Could you check a few things on this model? Use its own coordinates, in mm. A direction names the side the tool comes from. Round coordinates to 2 decimals unless told otherwise and drop trailing zeros. Write each loop counter-clockwise with the first axis right and the second up, starting at its lowest first coordinate (ties: lowest second). Pieces come first, ordered by that corner, then holes. Notation, with made-up numbers: (-8.75, 45.5) -> (29.25, 45.5) arc R34 cw to (29.25, 77.5) -> close; hole circle Ø7 at (62, 23.5). An arc over 180 degrees is marked (long way). Answer as CSV lines item,"result". Start each with the question number.
Q1. If I drill on line 1 (Y direction, x = 3.25, z = -2.5); line 2 (Y direction, x = -1.5, z = -2); line 3 (X direction, y = 4.5, z = 4), over which ranges is the centre line in solid material (lowest first)? Write a range as [from, to].
Q2. Imagine slicing it at A-A on z = 0. Please give me the cut outline in (x, y).
Q3. Imagine slicing it at B-B on x = 0. Please give me the cut outline in (y, z).
Q4. Imagine slicing it at C-C on y = 16.5. Please give me the cut outline in (x, z), and give its area (3 significant figures).
Q5. Will these pins go through, and if not, where does the flat tip stop? pin 1 Ø1.5 at (x, y) = (-1.5, 10) entering from -Z; pin 2 Ø0.5 at (x, z) = (0.5, -2.5) entering from +Y; pin 3 Ø2 at (x, y) = (-0.5, 12.5) entering from +Z.
Q6. For faces 1 (the flat face through (-1.054, -9.855, -1.101)), 2 (the flat face through (0, 10.947, -2)), 3 (the flat face through (1.054, -9.855, 1.101)), 4 (the cylindrical face through (1.99, -9.85, -1.96)), which set-ups out of +Z, -Z, +X, -X, +Y, -Y let a thin tool reach every point of the face, with its end or its side?
Autodesk Inventor part; units mm, degrees
ref_plane "at518_XY" through (0, 3.4925, 0) normal (0, -1, 0) x (1, 0, 0)
ref_plane "at518_YZ" through (0, 3.4925, 0) normal (1, 0, 0) x (0, 0, 1)
ref_plane "at518_ZX" through (0, 3.4925, 0) normal (0, 0, 1) x (0, -1, 0)
sketch "Sketch_2" plane through (0, 0, 0) normal (1, 0, 0) x (0, 1, 0)
  line L0 (0, 0) -> (20.0152, 0)
  line L1 (20.0152, 0) -> (20.0152, -2.7432)
  line L2 (20.0152, -2.7432) -> (19.7612, -2.9972)
  line L3 (19.7612, -2.9972) -> (10.0076, -2.9972)
  line L4 (10.0076, -2.9972) -> (10.0076, -4.54)
  line L5 (10.0076, -4.54) -> (9.5476, -5)
  line L6 (9.5476, -5) -> (0, -5)
  line L7 (0, -5) -> (0, 0)
  line L8 (0, 0) -> (20.0152, 0)
revolve "Revolution1" add sketch "Sketch_2" angle 360 about axis through (0, 0, 0) along (0, -1, 0)
thread "Thread1"
sketch "Sketch_3" plane through (0, 20.0152, 0) normal (0, 1, 0) x (1, 0, 0)
  line L0 (-2.6517, 1.397) -> (2.6517, 1.397)
  arc A0 (2.6517, 1.397) -> (-2.6517, 1.397) centre (0, 0) ccw
extrude "Extrusion1" cut sketch "Sketch_3" against normal blind 9.0678
sketch "Sketch_5" plane through (0, 0, 0) normal (0, 1, 0) x (-1, 0, 0)
  arc A0 (2.7335, 0.5782) -> (0.5782, 2.7335) centre (0, 0) ccw
  line L0 (0.5782, 2.7335) -> (-2.7335, -0.5782)
  arc A1 (-2.7335, -0.5782) -> (-0.5782, -2.7335) centre (0, 0) ccw
  line L1 (-0.5782, -2.7335) -> (2.7335, 0.5782)
extrude "Extrusion2" add sketch "Sketch_5" against normal blind 19.9898
sketch "Sketch_10" plane through (0, 0, 0) normal (0, 1, 0) x (-1, 0, 0)
  line L0 (4.0411, -3.5023) -> (3.5023, -2.9635)
  line L1 (3.5023, -2.9635) -> (2.9635, -3.5023)
  line L2 (2.9635, -3.5023) -> (3.5023, -4.0411)
  line L3 (3.5023, -4.0411) -> (4.0411, -3.5023)
extrude "Extrusion3" cut sketch "Sketch_10" along normal blind 25.4
ref_plane "at518_XY" through (0, 3.4925, 0) normal (0, -1, 0) x (1, 0, 0)
ref_plane "at518_YZ" through (0, 3.4925, 0) normal (1, 0, 0) x (0, 0, 1)
ref_plane "at518_ZX" through (0, 3.4925, 0) normal (0, 0, 1) x (0, -1, 0)
ref_plane "at520_XY" through (0, 2.5019, 0) normal (0, -1, 0) x (1, 0, 0)
ref_plane "at520_YZ" through (0, 2.5019, 0) normal (1, 0, 0) x (0, 0, 1)
ref_plane "at520_ZX" through (0, 2.5019, 0) normal (0, 0, 1) x (0, -1, 0)
ref_plane "at526_a_XY" through (0, 1.0033, 0) normal (0, -1, 0) x (1, 0, 0)
ref_plane "at526_a_YZ" through (0, 1.0033, 0) normal (1, 0, 0) x (0, 0, 1)
ref_plane "at526_a_ZX" through (0, 1.0033, 0) normal (0, 0, 1) x (0, -1, 0)
ref_plane "at526_b_XY" through (0, 4.9911, 0) normal (0, -1, 0) x (1, 0, 0)
ref_plane "at526_b_YZ" through (0, 4.9911, 0) normal (1, 0, 0) x (0, 0, 1)
ref_plane "at526_b_ZX" through (0, 4.9911, 0) normal (0, 0, 1) x (0, -1, 0)
ref_plane "to_body_XY" through (0, 0, 0) normal (0, 1, 0) x (1, 0, 0)
ref_plane "to_body_YZ" through (0, 0, 0) normal (1, 0, 0) x (0, 0, -1)
ref_plane "to_body_ZX" through (0, 0, 0) normal (0, 0, -1) x (0, 1, 0)
properties part number "HS13Z-D-shaft"
Checks:
1,line 1,"[0, 10.01]"
1,line 2,"[0, 10.95]"
1,line 3,"[-3, 3]"
2,outline,"(-5, 0) -> (-2.16, 0) -> (-2.16, -19.99) -> (2.16, -19.99) -> (2.16, 0) -> (5, 0) -> (5, 9.55) -> (4.54, 10.01) -> (3, 10.01) -> (3, 19.76) -> (2.74, 20.02) -> (-2.74, 20.02) -> (-3, 19.76) -> (-3, 10.01) -> (-4.54, 10.01) -> (-5, 9.55) -> close"
3,outline,"(-19.99, -2.16) -> (0, -2.16) -> (0, -5) -> (9.55, -5) -> (10.01, -4.54) -> (10.01, -3) -> (10.95, -3) -> (10.95, -1.4) -> (20.02, -1.4) -> (20.02, 2.74) -> (19.76, 3) -> (10.01, 3) -> (10.01, 4.54) -> (9.55, 5) -> (0, 5) -> (0, 2.16) -> (-19.99, 2.16) -> close"
4,outline,"(-2.65, -1.4) -> (2.65, -1.4) arc R3 ccw (long way) to start"
4,area,"22.2 mm^2"
5,pin 1,"z = -4.92"
5,pin 2,"y = 10.95"
5,pin 3,"z = 3"
6,face 1,"-Z, -X, -Y"
6,face 2,"-Z, +X, -X, +Y"
6,face 3,"+Z, +X, -Y"
6,face 4,"-Z, +X, -Y"
